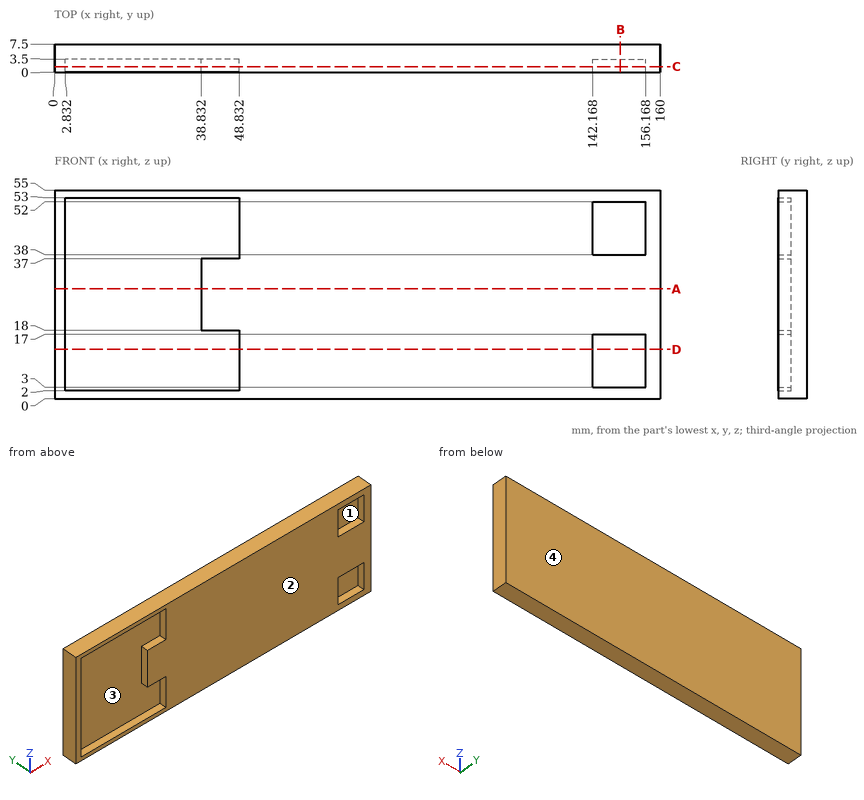
Answer from the drawing. Dimensions are ordinates in mm from the lowest x, y and z of the part. A direction names the side the tool comes from. Give positions to 0.01 mm unless a question says otherwise; leave off trailing zeros. Order: outer loops, then holes, each group sorted by start corner. A loop starts at its lowest first (then second) coordinate and runs counter-clockwise, first axis right, second up. Notation, with made-up numbers: (-1.75, 5) -> (38.25, 5) arc R8 cw to (38.25, 10) -> close; hole circle Ø4 at (82, -34). An arc over 180 degrees is marked (long way). Answer as a JSON object with one key per item and string values. Group by question number.
1. Flat-ended cylindrical pins translate along their axes: pin 1 Ø3 at (x, y) = (146.5, 2) entering from -Z; pin 2 Ø10 at (x, z) = (17, 18) entering from -Y. Find the tip coordinate at first contact, or state that the pin passes through.
2. Consider line 1 along Z through (x, y) = (39, 3.25); line 2 along X through (y, z) = (2.5, 22.5); line 3 along Y through (x, z) = (151.5, 48). Determine where each line is inside the solid, lowest interval first. Write a range as [from, to].
3. The mould has two halves that part along Z. Classify the marked faces 3 and 4: released by +Z, released by -Z, zero draft, split by the parting line, or undercut.
4. A tool of negligible diameter and unlimited length cuts with its end or side. For the marked faces 1 and 2, from which of +Z, -Z, +X, -X, +Y, -Y can it reach the whole face along a straight path? Write none if from no direction.
5. Section A-A on z = 29 is taken. Determine the outline of the cut face in (x, y).
6. Section B-B on x = 149.5 is taken. Determine the outline of the cut face in (y, z).
7. Section D-D on z = 13 is taken. Determine the outline of the cut face in (x, y).
8. Section C-C on y = 1.5 is taken. Determine the outline of the cut face in (x, z), plus the area to 3 significant figures.
Result sheet:
{
 "1": {"pin 1": "stops at z = 0", "pin 2": "stops at y = 3.5"},
 "2": {"line 1": "z = [0, 2], [18, 37], [53, 55]", "line 2": "x = [0, 2.83], [38.83, 160]", "line 3": "y = [3.5, 7.5]"},
 "3": {"face 3": "undercut", "face 4": "zero draft"},
 "4": {"face 1": "-Y", "face 2": "+Z, -Z, +X, -X, -Y"},
 "5": {"outline": "(0, 0) -> (2.83, 0) -> (2.83, 3.5) -> (38.83, 3.5) -> (38.83, 0) -> (160, 0) -> (160, 7.5) -> (0, 7.5) -> close"},
 "6": {"outline": "(0, 0) -> (7.5, 0) -> (7.5, 55) -> (0, 55) -> (0, 52) -> (3.5, 52) -> (3.5, 38) -> (0, 38) -> (0, 17) -> (3.5, 17) -> (3.5, 3) -> (0, 3) -> close"},
 "7": {"outline": "(0, 0) -> (2.83, 0) -> (2.83, 3.5) -> (48.83, 3.5) -> (48.83, 0) -> (142.17, 0) -> (142.17, 3.5) -> (156.17, 3.5) -> (156.17, 0) -> (160, 0) -> (160, 7.5) -> (0, 7.5) -> close"},
 "8": {"outline": "(0, 0) -> (160, 0) -> (160, 55) -> (0, 55) -> close; hole (2.83, 2) -> (48.83, 2) -> (48.83, 18) -> (38.83, 18) -> (38.83, 37) -> (48.83, 37) -> (48.83, 53) -> (2.83, 53) -> close; hole (142.17, 3) -> (156.17, 3) -> (156.17, 17) -> (142.17, 17) -> close; hole (142.17, 38) -> (156.17, 38) -> (156.17, 52) -> (142.17, 52) -> close", "area": "6,250 mm^2"}
}
